Verification items for the finished model (mm, model axes). A direction names the side the tool comes from. Coordinates: 2 decimals unless noted, no trailing zeros. Order: outer loops, then holes, each group sorted by start corner. A loop starts at its lowest first (then second) coordinate and runs counter-clockwise, first axis right, second up. Notation, with made-up numbers: (17, 87) -> (74, 87) arc R11 cw to (74, 102) -> close; hole circle Ø10 at (18.5, 88). An arc over 180 degrees is marked (long way). Write each question's results on one line, items separated by ' | '. Start each with the question number.
(1) Cross-section at B-B on z = -4. Enter the section's corners in (x, y).
(2) Set-up check for faces 1 (the cylindrical face through (-4.5, 2.4, 2.5)), 2 (the flat face through (3, -3, -7.6)), 3 (the flat face through (2, 5, -5.9)): record each of +Z, -Z, +X, -X, +Y, -Y from which the full face is reachable in a straight line by a thin tool's end or side.
(3) Cross-section at C-C on y = 3.25. Enter the section's corners in (x, z), and give its area (3 significant figures).
(4) Draft check along Y on faces 4 (the cylindrical face through (-0.228, -9.735, -4.174)), 5 (the flat face through (2, 5, -2.4)), 6 (the cylindrical face through (-4.5, 2.4, -6.8)). Enter one of: +Y half, -Y half, draft (parallel to the pull), parting line (faces both ways), or undercut.
(5) Cross-section at A-A on y = 0. Enter the section's corners in (x, z).
(6) Thickness scan on probe 1 along X at (y, z) = (0, -3.5); probe 2 along X at (y, z) = (0, -2.25); probe 3 along Z at (x, y) = (0.25, 10). Record the ranges inside material, lowest first. Write a range as [from, to].
(7) Go/stop test with flat-tipped pins: pin 1 (6 mm diameter, centred on x = 8, z = -2.5, fed in from +Y); pin 2 (4 mm diameter, centred on x = 0, y = -8, fed in from -Z); pin 3 (4 mm diameter, centred on y = -5.5, z = -3.5, fed in from +X); pin 4 (2 mm diameter, centred on x = 8, y = 0, fed in from +Z). Record where each tip stops, or that it passes through.
(8) Cross-section at D-D on x = 8. Enter the section's corners in (y, z), and give its area (3 significant figures).
Autodesk Inventor part; units mm, degrees
ref_plane "YZ Plane" through (0, 0, 0) normal (1, 0, 0) x (0, 1, 0)
ref_plane "XZ Plane" through (0, 0, 0) normal (0, 1, 0) x (-1, 0, 0)
ref_plane "XY Plane" through (0, 0, 0) normal (0, 0, 1) x (1, 0, 0)
sketch "Sketch1" plane through (0, 0, 0) normal (1, 0, 0) x (0, 1, 0)
  line L0 (5.1, -7.6) -> (0, -7.6)
  line L1 (0, -7.6) -> (0, 7.6) construction
  line L2 (0, 7.6) -> (5.1, 7.6)
  line L3 (5.1, 7.6) -> (5.1, -7.6)
  line L4 (11, -2.4) -> (5.1, -2.4)
  line L5 (5.1, -2.4) -> (5.1, -5.9)
  line L6 (5.1, -5.9) -> (11, -5.9)
  line L7 (11, -5.9) -> (11, -2.4)
  line L8 (4, 7.6) -> (4, -7.6)
  point P0 (0, 0)
  point P1 (0, 0)
  dimension "d0" = 5.1
  dimension "d1" = 15.2
  dimension "d2" = 3.5
  dimension "d3" = 10
  dimension "d4" = 11
  dimension "d5" = 0
  dimension "d6" = 4
revolve "Revolution1" add sketch "Sketch1" angle 360 about axis through (0, 0, -7.6) along (0, 0, 1)
sketch "Sketch2" plane through (0, 0, -5.9) normal (0, 0, -1) x (-1, 0, 0)
  circle A0 centre (0, 0) radius 11
  circle A1 centre (0, 0) radius 5.1
  circle A2 centre (0, 8) radius 1.75
  point P0 (0, 0)
  dimension "d8" = 3.5
  dimension "d9" = 8
extrude "Extrusion1" cut sketch "Sketch2" against normal blind 4 contours A2
pattern_circular "Circular Pattern1" count 4 over 360 about axis through (0, 0, -10) along (0, 0, 1) of "Extrusion1"
properties part number "LeadScrewNut"
Results are:
1) outline: circle Ø22 at (0, 0); hole circle Ø3.5 at (-8, 0); hole circle Ø8 at (0, 0); hole circle Ø3.5 at (0, -8); hole circle Ø3.5 at (0, 8); hole circle Ø3.5 at (8, 0)
2) face 1: +Z | face 2: -Z, +X, -X, +Y, -Y | face 3: -Z
3) outline: (-10.51, -5.9) -> (-3.93, -5.9) -> (-3.93, -7.6) -> (-2.33, -7.6) -> (-2.33, 7.6) -> (-3.93, 7.6) -> (-3.93, -2.4) -> (-10.51, -2.4) -> close; (2.33, -7.6) -> (3.93, -7.6) -> (3.93, -5.9) -> (10.51, -5.9) -> (10.51, -2.4) -> (3.93, -2.4) -> (3.93, 7.6) -> (2.33, 7.6) -> close | area: 94.6 mm2
4) face 4: undercut | face 5: draft | face 6: parting line
5) outline: (-11, -5.9) -> (-9.75, -5.9) -> (-9.75, -2.4) -> (-11, -2.4) -> close; (-6.25, -5.9) -> (-5.1, -5.9) -> (-5.1, -7.6) -> (-4, -7.6) -> (-4, 7.6) -> (-5.1, 7.6) -> (-5.1, -2.4) -> (-6.25, -2.4) -> close; (4, -7.6) -> (5.1, -7.6) -> (5.1, -5.9) -> (6.25, -5.9) -> (6.25, -2.4) -> (5.1, -2.4) -> (5.1, 7.6) -> (4, 7.6) -> close; (9.75, -5.9) -> (11, -5.9) -> (11, -2.4) -> (9.75, -2.4) -> close
6) probe 1: x = [-11, -9.75], [-6.25, -4], [4, 6.25], [9.75, 11] | probe 2: x = [-5.1, -4], [4, 5.1] | probe 3: z = [-5.9, -2.4]
7) pin 1: stops at y = 9.8 | pin 2: stops at z = -5.9 | pin 3: stops at x = 10.43 | pin 4: passes through
8) outline: (-7.55, -5.9) -> (-1.75, -5.9) -> (-1.75, -2.4) -> (-7.55, -2.4) -> close; (1.75, -5.9) -> (7.55, -5.9) -> (7.55, -2.4) -> (1.75, -2.4) -> close | area: 40.6 mm2
